from build123d import *

# Parameters (mm, degrees)
EXTRUDE_1_DEPTH     = 2
SKETCH_2_R          = 2.575
SKETCH_2_R_2        = 0.85
EXTRUDE_2_DEPTH     = 1.5
SKETCH_3_R          = 1.55
CUT_EXTRUDE_1_DEPTH = 0.3
CUT_EXTRUDE_2_DEPTH = 2.2


with BuildPart() as part:
    # ｽｹｯﾁ1 → ﾎﾞｽ - 押し出し1 (new body)
    with BuildSketch(Plane(origin=(0, 0, 0), x_dir=(1, 0, 0), z_dir=(0, 1, 0))):
        with BuildLine():
            Line((2.65, 4.705050478), (2.65, 2.65))
            Line((2.65, 2.65), (4.705050478, 2.65))
            ThreePointArc((4.705050478, 2.65), (5.4, 0), (4.705050478, -2.65))
            Line((4.705050478, -2.65), (2.65, -2.65))
            Line((2.65, -2.65), (2.65, -4.705050478))
            ThreePointArc((2.65, -4.705050478), (0, -5.4), (-2.65, -4.705050478))
            Line((-2.65, -4.705050478), (-2.65, -2.65))
            Line((-2.65, -2.65), (-4.705050478, -2.65))
            ThreePointArc((-4.705050478, -2.65), (-5.4, 0), (-4.705050478, 2.65))
            Line((-4.705050478, 2.65), (-2.65, 2.65))
            Line((-2.65, 2.65), (-2.65, 4.705050478))
            ThreePointArc((-2.65, 4.705050478), (0, 5.4), (2.65, 4.705050478))
        make_face()
    extrude(amount=EXTRUDE_1_DEPTH)

    # ｽｹｯﾁ2 → ﾎﾞｽ - 押し出し2 (add)
    with BuildSketch(Plane.XZ):
        with Locations(Location((0, 0, 0), (0, 0, 90))):
            Circle(SKETCH_2_R)
        with Locations(Location((0, 0, 0), (0, 0, 270))):
            Circle(SKETCH_2_R_2, mode=Mode.SUBTRACT)
    extrude(amount=EXTRUDE_2_DEPTH)

    # ｽｹｯﾁ3 → ｶｯﾄ - 押し出し1 (cut)
    with BuildSketch(Plane.XZ.offset(1.5)):
        with Locations(Location((0, 0, 0), (0, 0, 270))):
            Circle(SKETCH_3_R)
    extrude(amount=-CUT_EXTRUDE_1_DEPTH, mode=Mode.SUBTRACT)

    # ｽｹｯﾁ4 → ｶｯﾄ - 押し出し2 (cut)
    with BuildSketch(Plane(origin=(0, 2, 0), x_dir=(1, 0, 0), z_dir=(0, 1, 0))):
        Polygon((0, 1.6), (0.437016815, 2.056002469), (0.650778629, 1.461672732), (1.235486269, 1.700500964), (1.189031721, 1.07060897), (1.820328922, 1.050967393), (1.521690426, 0.494427191), (2.090420168, 0.219712013), (1.591235033, -0.167245541), (1.999058776, -0.64953357), (1.385640646, -0.8), (1.56204196, -1.406468898), (0.940456404, -1.294427191), (0.854933899, -1.920212977), (0.332658705, -1.565036161), (0, -2.101934787), (-0.332658705, -1.565036161), (-0.854933899, -1.920212977), (-0.940456404, -1.294427191), (-1.56204196, -1.406468898), (-1.385640646, -0.8), (-1.999058776, -0.64953357), (-1.591235033, -0.167245541), (-2.090420168, 0.219712013), (-1.521690426, 0.494427191), (-1.820328922, 1.050967393), (-1.189031721, 1.07060897), (-1.235486269, 1.700500964), (-0.650778629, 1.461672732), (-0.437016815, 2.056002469), align=None)
    extrude(amount=-CUT_EXTRUDE_2_DEPTH, mode=Mode.SUBTRACT)


solid = part.part
The listing builds one solid part. Answer for the finished solid, in the listing's coordinates (mm). A direction names the side the tool comes from. Coordinates: 2 decimals unless noted, no trailing zeros. Write each loop counter-clockwise with the first axis right and the second up, starting at its lowest first coordinate (ties: lowest second). Pieces come first, ordered by that corner, then holes. Notation, with made-up numbers: (-39, -21.75) - (-10, -21.75) arc R6 ccw to (-10, -13.75) - close; hole circle Ø11 at (16.5, 39). An arc over 180 degrees is marked (long way). Answer as CSV lines item,"result".
1. Find section B-B (y = -0.5). Give the vertices of the cut face in (x, z) (3 decimals).
Computed values:
outline,"circle Ø5.15 at (0, 0); hole circle Ø1.7 at (0, 0)"
2. A tool of negligible diameter and unlimited length cuts with its end or side. For faces 4 (the flat face through (-2.65, 1, 4)), 5 (the flat face through (-4, 1, -2.65)), 6 (the flat face through (-1, -0.2, 0)), from which of +Z, -Z, +X, -X, +Y, -Y can it reach the whole face along a straight path? Write none if from no direction.
Computed values:
face 4,"+Z, -X, +Y, -Y"
face 5,"-Z, -X, +Y, -Y"
face 6,"+Y"
3. Find section D-D (z = 4.5). Give the vertices of the cut face in (x, y), plus the area to 3 significant figures.
Computed values:
outline,"(-2.65, 0) - (2.65, 0) - (2.65, 2) - (-2.65, 2) - close"
area,"10.6 mm²"
4. Find section C-C (x = 4.25). Give the vertices of the cut face in (y, z), plus the area to 3 significant figures.
Computed values:
outline,"(0, -2.65) - (2, -2.65) - (2, 2.65) - (0, 2.65) - close"
area,"10.6 mm²"
5. Straight lines are drawn through the part: line 1 (X direction, y = -1.3, z = 0) (3 decimals); line 2 (X direction, y = -0.8, z = 0) (3 decimals); line 3 (Y direction, x = -3.5, z = 2). For each, find the intervals that lie inside material, in ascending order. Write a range as [from, to].
Computed values:
line 1,"x = [-2.575, -1.55], [1.55, 2.575]"
line 2,"x = [-2.575, -0.85], [0.85, 2.575]"
line 3,"y = [0, 2]"
6. Find section A-A (z = 0). Give the vertices of the cut face in (x, y) (3 decimals), plus the area to 3 significant figures.
Computed values:
outline,"(-5.4, 0) - (-2.575, 0) - (-2.575, -1.5) - (-1.55, -1.5) - (-1.55, -1.2) - (-0.85, -1.2) - (-0.85, -0.2) - (-1.807, -0.2) - (-1.807, 2) - (-5.4, 2) - close; (0.85, -1.2) - (1.55, -1.2) - (1.55, -1.5) - (2.575, -1.5) - (2.575, 0) - (5.4, 0) - (5.4, 2) - (1.807, 2) - (1.807, -0.2) - (0.85, -0.2) - close"
area,"18.7 mm²"
7. Given P1, Ø1, axis at y = 1, z = -3.5, coming from the +X side; P2, Ø1, axis at y = 0.5, z = -1.5, coming from the -X side; P3, Ø1.6, axis at y = 1, z = 3.5, coming from the -X side, each flat-ended and moving along its own axis, determine where each tip first touches the part or whether it passes through.
Computed values:
P1,"stops at x = 2.65"
P2,"stops at x = -5.31"
P3,"stops at x = -2.65"
8. Determine the mould class of faces 1 (the flat face through (0, -1.2, -1)), 2 (the flat face through (4, 1, 2.65)), 3 (the cylindrical face through (0, 1, 5.4)) for opening direction X: +X half, -X half, draft (parallel to the pull), parting line (faces both ways), or undercut.
Computed values:
face 1,"undercut"
face 2,"draft"
face 3,"parting line"
